```python
from build123d import *

# Parameters (mm, degrees)
FLANGE_HOLES_D    = 2.8702
DOWEL_HOLES_D     = 4.7625
DOWEL_HOLES_DEPTH = 6.35
DOWEL_HOLES_TIP   = 1.430799349
FILLET1_R         = 8.89
CHAMFER1_SIZE     = 2.141545552
CHAMFER1_SIZE_2   = 2.54


with BuildPart() as part:
    # Sketch2 → Main Structure (revolve)
    with BuildSketch(Plane.XY, mode=Mode.PRIVATE) as main_structure_sk:
        Polygon((0, 20.583496156), (0, 56.388), (9.525, 56.388), (9.525, 16.256), (66.806461084, 16.256), (139.7, 31.75), (139.7, 29.592458901), (60.325, 12.720781818), (60.325, 14.351), (10.795, 14.351), align=None)
    revolve(main_structure_sk.sketch.rotate(Axis((0, 0, 0), (1, 0, 0)), 90), axis=Axis((0, 0, 0), (1, 0, 0)))

    # Flange Holes (through all)
    with Locations(Plane.ZY):
        with Locations((0, -51.6255), (-25.81275, -44.708994483), (-44.708994483, -25.81275), (-51.6255, 0), (-44.708994483, 25.81275), (-25.81275, 44.708994483), (0, 51.6255), (25.81275, 44.708994483), (44.708994483, 25.81275), (51.6255, 0), (44.708994483, -25.81275), (25.81275, -44.708994483)):
            Hole(FLANGE_HOLES_D / 2)

    # Dowel Holes
    with Locations(Plane.ZY):
        with Locations((49.866403745, -13.361662613), (-49.866403745, 13.361662613)):
            Hole(DOWEL_HOLES_D / 2, depth=DOWEL_HOLES_DEPTH)
            with Locations((0, 0, -(DOWEL_HOLES_DEPTH + DOWEL_HOLES_TIP / 2))):  # 118° drill point
                Cone(0, DOWEL_HOLES_D / 2, DOWEL_HOLES_TIP, mode=Mode.SUBTRACT)

    # Fillet1
    fillet1_edges = [part.edges().sort_by_distance(p)[0] for p in [
        (9.525, 0, -16.256),
    ]]
    fillet(fillet1_edges, radius=FILLET1_R)

    # Sketch13 → Cut-Revolve1 (revolve, cut)
    with BuildSketch(Plane(origin=(0, 0, 0), x_dir=(1, 0, 0), z_dir=(0, 1, 0)), mode=Mode.PRIVATE) as cut_revolve1_sk:
        Polygon((0, 38.1), (3.33331808, 0), (0, 0), align=None)
    revolve(cut_revolve1_sk.sketch.rotate(Axis((3.33331808, 0, 0), (-1, 0, 0)), 180), axis=Axis((3.33331808, 0, 0), (-1, 0, 0)), mode=Mode.SUBTRACT)

    # Chamfer1
    # the kernel refuses this chamfer: 2.54, 2.141545552 mm, written as the material it takes off along each edge
    with BuildSketch(Plane(origin=(139.7, 0, 0), x_dir=(0, 0, 1), z_dir=(0, 1, 0))) as chamfer1_piece_1:
        Polygon((31.75 - CHAMFER1_SIZE * 0.207911690799, -CHAMFER1_SIZE * 0.978147600645), (31.75 - CHAMFER1_SIZE_2, 0), (31.75, 0), align=None)
    revolve(axis=Axis((139.7, 0, 0), (1, 0, 0)), mode=Mode.SUBTRACT)


solid = part.part
```
Here's how the part is built. I have some questions about the finished solid (model axes, mm). A direction names the side the tool comes from. Coordinates: 2 decimals unless noted, no trailing zeros. Loops run counter-clockwise (first coordinate to the right, second up) from the corner with the lowest first, then second, coordinate; pieces in that order, holes last. Notation, with made-up numbers: (7, 51) - (20, 51) arc R29 ccw to (20, 85) - close; hole circle Ø9 at (-25, -15). An arc over 180 degrees is marked (long way). Return JSON: item names as keys, results as strings. Group by question number.
Item 1: We'd pull the mould along Y, two halves only. Please class faces 4 (the face through (35.213, 12.732, 6.622)), 5 (the face through (0, 12, -37)), 6 (the face through (4.829, 50.026, 26.02)): +Y half, -Y half, draft (parallel to the pull), parting line (faces both ways), or undercut.
Item 2: Will these pins go through, and if not, where does the flat tip stop? P1, Ø1, axis at x = 24, y = -12.5, coming from the +Z side; P2, Ø12, axis at x = 56.5, y = -9.5, coming from the -Z side; P3, Ø7.5, axis at y = -13.36, z = 49.87, coming from the +X side (3 decimals).
Item 3: If we section it at B-B on x = 13.5: Write out the boundary of the cut face in (y, z), and give its area (3 significant figures).
Item 4: On a 3-axis mill with a long thin cutter (end or side, diameter ignored), from which of +Z, -Z, +X, -X, +Y, -Y can I reach the whole of each face in a straight line? I mean faces 1 (the face through (99.3, 12.78, -16.67)), 2 (the face through (3.219, 12.45, -52.066)), 3 (the face through (42.95, 15.87, -3.52)). Say none if no direction works.
Item 5: I need wall thicknesses on line 1 (Z direction, x = 41, y = -0.5); line 2 (Y direction, x = 6.75, z = 0); line 3 (Z direction, x = 120.5, y = 0.5). Which ranges of each line are inside material? Lowest first, please. Write a range as from..to.
Item 6: If we section it at A-A on x = 38: Write out the boundary of the cut face in (y, z).
Calculated:
{
 "1": {"face 4": "undercut", "face 5": "draft", "face 6": "parting line"},
 "2": {"P1": "stops at z = 10.97", "P2": "stops at z = -15.87", "P3": "stops at x = 9.525"},
 "3": {"outline": "circle Ø35.48 at (0, 0); hole circle Ø28.7 at (0, 0)", "area": "341 mm^2"},
 "4": {"face 1": "+X", "face 2": "-X", "face 3": "none"},
 "5": {"line 1": "z = -16.25..-14.34, 14.34..16.25", "line 2": "y = -56.39..-53.06, -50.19..-16.69, 16.69..50.19, 53.06..56.39", "line 3": "z = -27.66..-25.51, 25.51..27.66"},
 "6": {"outline": "circle Ø32.51 at (0, 0); hole circle Ø28.7 at (0, 0)"}
}
